Read the model definition and answer for the solid it produces. Units are mm, in the model's axes. Face numbers are marked on the shaded views. A direction names the side the tool comes from. Round coordinates to 2 decimals unless told otherwise and drop trailing zeros. Write each loop counter-clockwise with the first axis right and the second up, starting at its lowest first coordinate (ties: lowest second). Pieces come first, ordered by that corner, then holes. Notation, with made-up numbers: (43, 83) -> (68, 83) arc R26 ccw to (68, 105) -> close; hole circle Ø6 at (-15.5, 24.5). An arc over 180 degrees is marked (long way). Return JSON: item names as keys, results as strings.
Autodesk Inventor part; units mm, degrees
ref_plane "Work Plane1" through (0, 0, 0) normal (0, 0, 1) x (1, 0, 0)
ref_plane "YZ Plane" through (0, 0, 0) normal (1, 0, 0) x (0, 1, 0)
ref_plane "XZ Plane" through (0, 0, 0) normal (0, 1, 0) x (-1, 0, 0)
sketch "Sketch1" plane through (0, 0, 0) normal (0, 0, 1) x (1, 0, 0)
  circle A0 centre (0, 0) radius 3.81
  circle A1 centre (0, 0) radius 4.4866
  circle A2 centre (0, 0) radius 20.32
  circle A3 centre (0, 0) radius 19.017
  dimension "d0" = 7.62
  dimension "d1" = 40.64
extrude "Extrusion1" add sketch "Sketch1" against normal blind 10
ref_plane "Work Plane1" through (0, 0, 0) normal (0, 0, 1) x (1, 0, 0)
sketch "Sketch2" plane through (0, 0, 0) normal (0, 0, 1) x (1, 0, 0)
  circle A0 centre (0, 0) radius 4.4866
  circle A1 centre (0, 0) radius 19.017
  line L0 (0, 4.4866) -> (4.4866, 18.4802)
  line L1 (3.4, 2.9274) -> (9.1521, 16.6699)
extrude "Extrusion2" add sketch "Sketch2" against normal blind 3 contours A0 L0 A1 L1 picked at (3.8455, 13.626)
pattern_circular "Circular Pattern1" count 6 over 360 about axis through (0, 0, 0) along (0, 0, -1) of "Extrusion2"
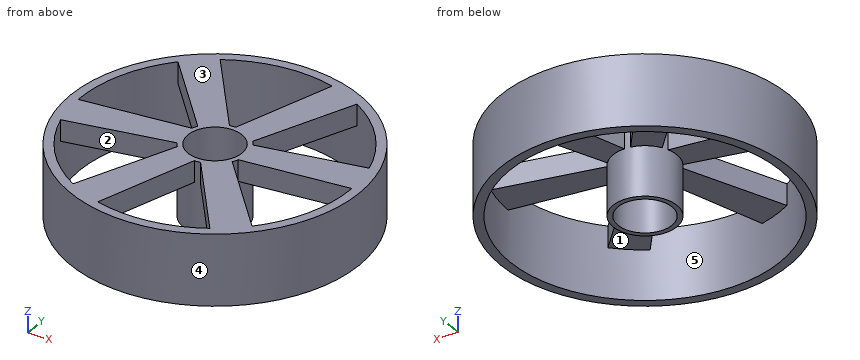
Item 1: For a pull along X with two mould halves and no side action, classify the marked faces 3, 4 and 5 as released by +X, released by -X, zero draft, split by the parting line, or undercut.
Worked answers:
{"face 3": "zero draft", "face 4": "split by the parting line", "face 5": "undercut"}
Item 2: Section B-B (x = 6) is taken. Give the vertices of the cut face in (y, z).
Worked answers:
{"outline": "(-19.41, -10) -> (-18.05, -10) -> (-18.05, 0) -> (-19.41, 0) -> close; (-11.19, -3) -> (-4.57, -3) -> (-4.57, 0) -> (-11.19, 0) -> close; (-1.26, -3) -> (2.7, -3) -> (2.7, 0) -> (-1.26, 0) -> close; (9.14, -3) -> (18.05, -3) -> (18.05, -10) -> (19.41, -10) -> (19.41, 0) -> (9.14, 0) -> close"}
Item 3: A tool of negligible diameter and unlimited length cuts with its end or side. For the marked faces 1 and 2, from which of +Z, -Z, +X, -X, +Y, -Y can it reach the whole face along a straight path? Write none if from no direction.
Worked answers:
{"face 1": "-Z", "face 2": "+Z, -Z"}
Item 4: Section A-A (z = -5.75) is taken. Give the vertices of the cut face in (x, y), then the cut area to 3 significant figures.
Worked answers:
{"outline": "circle Ø40.64 at (0, 0); circle Ø8.97 at (0, 0); hole circle Ø38.03 at (0, 0); hole circle Ø7.62 at (0, 0)", "area": "179 mm2"}
Item 5: Section C-C (y = 8) is taken. Give the vertices of the cut face in (x, z), then the cut area to 3 significant figures.
Worked answers:
{"outline": "(-18.68, -10) -> (-17.25, -10) -> (-17.25, 0) -> (-18.68, 0) -> close; (-9.11, -3) -> (-3.57, -3) -> (-3.57, 0) -> (-9.11, 0) -> close; (1.13, -3) -> (5.52, -3) -> (5.52, 0) -> (1.13, 0) -> close; (17.25, -10) -> (18.68, -10) -> (18.68, 0) -> (17.25, 0) -> close", "area": "58.3 mm2"}
Item 6: Straight lines are drawn through the part: L1, parallel to Y at x = 0, z = -7; L2, parallel to Y at x = 1, z = -5.75; L3, parallel to X at y = 15, z = -0.25. For each, find the intervals that lie inside material, in ascending order. Write a range as [from, to].
Worked answers:
{"L1": "y = [-20.32, -19.02], [-4.49, -3.81], [3.81, 4.49], [19.02, 20.32]", "L2": "y = [-20.3, -18.99], [-4.37, -3.68], [3.68, 4.37], [18.99, 20.3]", "L3": "x = [-13.71, -8.9], [3.37, 8.45], [11.69, 13.71]"}
Item 7: Section D-D (z = -2.5) is taken. Give the vertices of the cut face in (x, y), then the cut area to 3 significant figures.
Worked answers:
{"outline": "circle Ø40.64 at (0, 0); hole (-19.01, -0.41) -> (-4.24, 1.48) arc R4.49 cw to (-3.89, 2.24) -> (-13.76, 13.13) arc R19.02 ccw to start; hole (-18.25, -5.35) arc R19.02 ccw to (-9.15, -16.67) -> (-3.4, -2.93) arc R4.49 cw to (-3.89, -2.24) -> close; hole (-9.86, 16.26) -> (-0.84, 4.41) arc R4.49 cw to (0, 4.49) -> (4.49, 18.48) arc R19.02 ccw to start; hole (-4.49, -18.48) arc R19.02 ccw to (9.86, -16.26) -> (0.84, -4.41) arc R4.49 cw to (0, -4.49) -> close; hole circle Ø7.62 at (0, 0); hole (3.4, 2.93) arc R4.49 cw to (3.89, 2.24) -> (18.25, 5.35) arc R19.02 ccw to (9.15, 16.67) -> close; hole (3.89, -2.24) -> (13.76, -13.13) arc R19.02 ccw to (19.01, 0.41) -> (4.24, -1.48) arc R4.49 cw to start", "area": "563 mm2"}
Item 8: Flat-ended cylindrical pins translate along their axes: pin 1 (1.5 mm diameter, centred on y = -15.5, z = -3, fed in from +X); pin 2 (4.5 mm diameter, centred on x = 0, y = 0, fed in from +Z); pin 3 (2 mm diameter, centred on x = -13.5, y = -2.5, fed in from -Z); pin 4 (10 mm diameter, centred on x = 6.5, y = 12.5, fed in from -Z). Find the tip coordinate at first contact, or state that the pin passes through.
Worked answers:
{"pin 1": "stops at x = 13.98", "pin 2": "passes through", "pin 3": "stops at z = -3", "pin 4": "stops at z = -10"}
